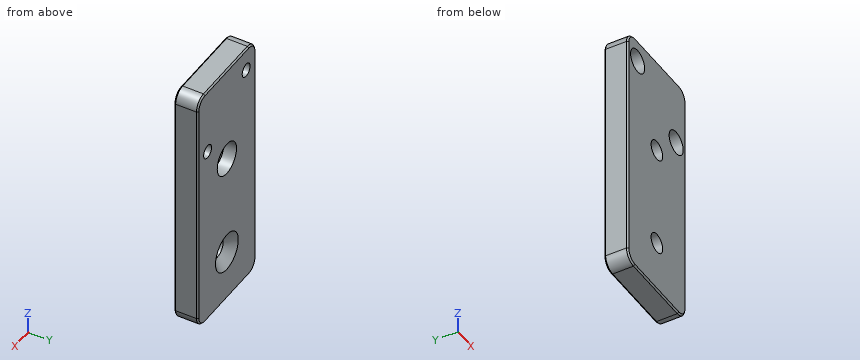
from build123d import *

# Parameters (mm, degrees)
SKETCH3_W           = 33
SKETCH3_H           = 86
SKETCH3_R           = 3.3
SKETCH3_R_2         = 2.25
BOSS_EXTRUDE2_DEPTH = 8
SKETCH4_R           = 5.5
CUT_EXTRUDE2_DEPTH  = 4.2
CHAMFER1_SIZE       = 3.2
SKETCH5_R           = 4
CUT_EXTRUDE3_DEPTH  = 4.4
FILLET1_R           = 4
CHAMFER2_SIZE       = 0.5


with BuildPart() as part:
    # Sketch3 → Boss-Extrude2 (new body)
    with BuildSketch(Plane(origin=(0, 0, 0), x_dir=(1, 0, 0), z_dir=(0, 1, 0))):
        Rectangle(SKETCH3_W, SKETCH3_H)
        with Locations((0, 25.5)):
            Circle(SKETCH3_R, mode=Mode.SUBTRACT)
        with Locations((0, -9.5)):
            Circle(SKETCH3_R, mode=Mode.SUBTRACT)
        with Locations((11, -20.3)):
            Circle(SKETCH3_R_2, mode=Mode.SUBTRACT)
        with Locations((-11, -35.3)):
            Circle(SKETCH3_R_2, mode=Mode.SUBTRACT)
    extrude(amount=BOSS_EXTRUDE2_DEPTH)

    # Sketch4 → Cut-Extrude2 (cut)
    with BuildSketch(Plane(origin=(0, 8, 0), x_dir=(1, 0, 0), z_dir=(0, 1, 0))):
        with Locations((0, -9.736308316)):
            Circle(SKETCH4_R)
    extrude(amount=-CUT_EXTRUDE2_DEPTH, mode=Mode.SUBTRACT)

    # Chamfer1
    chamfer1_edges = [part.edges().sort_by_distance(p)[0] for p in [
        (-3.3, 8, -25.5),
    ]]
    chamfer(chamfer1_edges, length=CHAMFER1_SIZE)

    # Sketch5 → Cut-Extrude3 (cut)
    with BuildSketch(Plane(origin=(0, 0, 0), x_dir=(-1, 0, 0), z_dir=(0, -1, 0))):
        with Locations((11, -35.3)):
            Circle(SKETCH5_R)
        with Locations((-11, -20.3)):
            Circle(SKETCH5_R)
    extrude(amount=-CUT_EXTRUDE3_DEPTH, mode=Mode.SUBTRACT)

    # Fillet1
    fillet1_edges = [part.edges().sort_by_distance(p)[0] for p in [
        (16.5, 4, 43),
        (-16.5, 4, 43),
        (-16.5, 4, -43),
        (16.5, 4, -43),
    ]]
    fillet(fillet1_edges, radius=FILLET1_R)

    # Chamfer2
    chamfer2_edges = [part.edges().sort_by_distance(p)[0] for p in [
        (16.5, 0, 0),
        (16.5, 8, 0),
        (0, 0, 43),
        (-16.5, 0, 0),
        (0, 0, -43),
        (15.328427125, 0, -41.828427125),
        (-15.328427125, 0, -41.828427125),
        (-15.328427125, 0, 41.828427125),
        (15.328427125, 0, 41.828427125),
        (0, 8, 43),
        (0, 8, -43),
        (-16.5, 8, 0),
        (15.328427125, 8, -41.828427125),
        (-15.328427125, 8, -41.828427125),
        (-15.328427125, 8, 41.828427125),
        (15.328427125, 8, 41.828427125),
    ]]
    chamfer(chamfer2_edges, length=CHAMFER2_SIZE)


solid = part.part
Design review of the part built by this model. Coordinates are the model's own, in mm. Round coordinates to 2 decimals unless told otherwise and drop trailing zeros. Write each loop counter-clockwise with the first axis right and the second up, starting at its lowest first coordinate (ties: lowest second). Pieces come first, ordered by that corner, then holes. Notation, with made-up numbers: (82, 7) - (133, 7) arc R34 ccw to (133, 42) - close; hole circle Ø11 at (82, -32). An arc over 180 degrees is marked (long way). Return JSON: item names as keys, results as strings. Group by question number.
Item 1: We need section C-C on z = 35.3. Write out the cut boundary in (x, y), and give its area (3 significant figures).
Item 2: We need section B-B on x = 0. Write out the cut boundary in (y, z), and give its area (3 significant figures).
Item 3: Insertion check: P1, Ø6.5, axis at x = -10.5, z = 35, coming from the -Y side; P2, Ø14.5, axis at x = 0, z = 9.74, coming from the +Y side. Each pin has a flat end and moves straight along its axis. Give the tip position at first contact, or say it passes through.
Item 4: For probe 1 along Z at (x, y) = (-11, 3.75); probe 2 along Z at (x, y) = (1, 4); probe 3 along Z at (x, y) = (11, 2.9), list the stretches that pass through material, from the lowest coordinate up. Write a range as [from, to].
Item 5: We need section A-A on x = -11. Write out the cut boundary in (y, z), and give its area (3 significant figures).
Item 6: We need section D-D on y = 3. Write out the cut boundary in (x, z).
Model answer:
{
 "1": {"outline": "(-16.5, 0.5) - (-16, 0) - (-15, 0) - (-15, 4.4) - (-13.25, 4.4) - (-13.25, 8) - (-16, 8) - (-16.5, 7.5) - close; (-8.75, 4.4) - (-7, 4.4) - (-7, 0) - (16, 0) - (16.5, 0.5) - (16.5, 7.5) - (16, 8) - (-8.75, 8) - close", "area": "212 mm²"},
 "2": {"outline": "(0, -42.5) - (0.5, -43) - (7.5, -43) - (8, -42.5) - (8, -32) - (4.8, -28.8) - (0, -28.8) - close; (0, -22.2) - (4.8, -22.2) - (8, -19) - (8, 4.24) - (3.8, 4.24) - (3.8, 6.2) - (0, 6.2) - close; (0, 12.8) - (3.8, 12.8) - (3.8, 15.24) - (8, 15.24) - (8, 42.5) - (7.5, 43) - (0.5, 43) - (0, 42.5) - close", "area": "553 mm²"},
 "3": {"P1": "stops at y = 4.4", "P2": "stops at y = 8"},
 "4": {"probe 1": "z = [-43, 31.3], [39.3, 43]", "probe 2": "z = [-43, -28.64], [-22.36, 4.33], [15.14, 43]", "probe 3": "z = [-43, 16.3], [24.3, 43]"},
 "5": {"outline": "(0, -42.5) - (0.5, -43) - (7.5, -43) - (8, -42.5) - (8, 33.05) - (4.4, 33.05) - (4.4, 31.3) - (0, 31.3) - close; (0, 39.3) - (4.4, 39.3) - (4.4, 37.55) - (8, 37.55) - (8, 42.5) - (7.5, 43) - (0.5, 43) - (0, 42.5) - close", "area": "636 mm²"},
 "6": {"outline": "(-16.5, -39) arc R4 ccw to (-12.5, -43) - (12.5, -43) arc R4 ccw to (16.5, -39) - (16.5, 39) arc R4 ccw to (12.5, 43) - (-12.5, 43) arc R4 ccw to (-16.5, 39) - close; hole circle Ø8 at (-11, 35.3); hole circle Ø6.6 at (0, -25.5); hole circle Ø6.6 at (0, 9.5); hole circle Ø8 at (11, 20.3)"}
}
